Could you check a few things on this model? Use its own coordinates, in mm. A direction names the side the tool comes from. Coordinates: 2 decimals unless noted, no trailing zeros. Order: outer loops, then holes, each group sorted by start corner. A loop starts at its lowest first (then second) coordinate and runs counter-clockwise, first axis right, second up. Notation, with made-up numbers: (13, 4.5) - (37, 4.5) arc R9 ccw to (37, 10.5) - close; hole circle Ø6 at (10, 47). An arc over 180 degrees is marked (long way). Answer as CSV lines item,"result". Start each with the question number.
1. Thinking about a two-plate mould opening in Z: for faces 1 (the face through (-3, 9.5, 3)), 2 (the face through (9.06, 3.94, 6.6)), which applies, released by +Z, released by -Z, zero draft, split by the parting line, or undercut?
2. I want a section at A-A, the plane x = 0. List the corners of the cut face in (y, z) for me, and give its area (3 significant figures).
3. For pin 1 (2.5 mm diameter, centred on x = -5.63, z = -4.95, fed in from +Y); pin 2 (1 mm diameter, centred on x = 5, y = 6, fed in from -Z); pin 3 (2 mm diameter, centred on y = 5, z = -10.5, fed in from -X); pin 4 (5 mm diameter, centred on x = 9, y = 6.5, fed in from +Z), each with a flat end and sliding along its axis, tell me the tip position at first contact or that it passes through.
4. I want a section at C-C, the plane y = 3. Count the separate pieces of the cut face and the enclosed holes in it, and give its area (3 significant figures).
5. I need wall thicknesses on probe 1 along X at (y, z) = (7, 0); probe 2 along Z at (x, y) = (10.75, 6); probe 3 along X at (y, z) = (8.5, -1). Which ranges of each line are inside material? Lowest first, please.
6. I want a section at B-B, the plane z = 0. List the corners of the cut face in (x, y) for me, and give its area (3 significant figures).
7. For faces 3 (the face through (-10, 3.94, 5.07)), 4 (the face through (11.21, 3.94, 0.02)), 5 (the face through (7.21, 4.68, -5.38)), which set-ups out of +Z, -Z, +X, -X, +Y, -Y let a thin tool reach every point of the face, with its end or its side?
from build123d import *

# Parameters (mm, degrees)
BOSS_EXTRUDE1_DEPTH = 8
SKETCH2_R           = 15
BOSS_EXTRUDE2_DEPTH = 1.5
SKETCH4_R           = 4
SKETCH4_R_2         = 1.5
CUT_EXTRUDE1_DEPTH  = 23


with BuildPart() as part:
    # Sketch1 → Boss-Extrude1 (new body)
    with BuildSketch(Plane(origin=(0, 0, 0), x_dir=(1, 0, 0), z_dir=(0, 1, 0))):
        with BuildLine():
            ThreePointArc((-2.619011045, 11.679969227), (-2.794341005, 11.639267947), (-2.969039138, 11.595934917))
            ThreePointArc((-2.969039138, 11.595934917), (-3.464080507, 10.661343548), (-4.413916411, 11.126465832))
            ThreePointArc((-4.413916411, 11.126465832), (-4.580720685, 11.058838004), (-4.746489215, 10.988709666))
            ThreePointArc((-4.746489215, 10.988709666), (-5.089233502, 9.988183136), (-6.100136506, 10.298991922))
            ThreePointArc((-6.100136506, 10.298991922), (-6.25430782, 10.206102767), (-6.407064974, 10.110905915))
            ThreePointArc((-6.407064974, 10.110905915), (-6.589072678, 9.069080507), (-7.636150994, 9.21792265))
            ThreePointArc((-7.636150994, 9.21792265), (-7.773893139, 9.102059408), (-7.909877531, 8.984138103))
            ThreePointArc((-7.909877531, 8.984138103), (-7.926667017, 7.926667017), (-8.984138103, 7.909877531))
            ThreePointArc((-8.984138103, 7.909877531), (-9.102059408, 7.773893139), (-9.21792265, 7.636150994))
            ThreePointArc((-9.21792265, 7.636150994), (-9.069080507, 6.589072678), (-10.110905915, 6.407064974))
            ThreePointArc((-10.110905915, 6.407064974), (-10.206102767, 6.25430782), (-10.298991922, 6.100136506))
            ThreePointArc((-10.298991922, 6.100136506), (-9.988183136, 5.089233502), (-10.988709666, 4.746489215))
            ThreePointArc((-10.988709666, 4.746489215), (-11.058838004, 4.580720685), (-11.126465832, 4.413916411))
            ThreePointArc((-11.126465832, 4.413916411), (-10.661343548, 3.464080507), (-11.595934917, 2.969039138))
            ThreePointArc((-11.595934917, 2.969039138), (-11.639267947, 2.794341005), (-11.679969227, 2.619011045))
            ThreePointArc((-11.679969227, 2.619011045), (-11.071986298, 1.753630353), (-11.917629765, 1.118481464))
            ThreePointArc((-11.917629765, 1.118481464), (-11.933100485, 0.939155376), (-11.945873016, 0.759616935))
            ThreePointArc((-11.945873016, 0.759616935), (-11.21, 0), (-11.945873016, -0.759616935))
            ThreePointArc((-11.945873016, -0.759616935), (-11.933100485, -0.939155376), (-11.917629765, -1.118481464))
            ThreePointArc((-11.917629765, -1.118481464), (-11.071986298, -1.753630353), (-11.679969227, -2.619011045))
            ThreePointArc((-11.679969227, -2.619011045), (-11.639267947, -2.794341005), (-11.595934917, -2.969039138))
            ThreePointArc((-11.595934917, -2.969039138), (-10.661343548, -3.464080507), (-11.126465832, -4.413916411))
            ThreePointArc((-11.126465832, -4.413916411), (-11.058838004, -4.580720685), (-10.988709666, -4.746489215))
            ThreePointArc((-10.988709666, -4.746489215), (-9.988183136, -5.089233502), (-10.298991922, -6.100136506))
            ThreePointArc((-10.298991922, -6.100136506), (-10.206102767, -6.25430782), (-10.110905915, -6.407064974))
            ThreePointArc((-10.110905915, -6.407064974), (-9.069080507, -6.589072678), (-9.21792265, -7.636150994))
            ThreePointArc((-9.21792265, -7.636150994), (-9.102059408, -7.773893139), (-8.984138103, -7.909877531))
            ThreePointArc((-8.984138103, -7.909877531), (-7.926667017, -7.926667017), (-7.909877531, -8.984138103))
            ThreePointArc((-7.909877531, -8.984138103), (-7.773893139, -9.102059408), (-7.636150994, -9.21792265))
            ThreePointArc((-7.636150994, -9.21792265), (-6.589072678, -9.069080507), (-6.407064974, -10.110905915))
            ThreePointArc((-6.407064974, -10.110905915), (-6.25430782, -10.206102767), (-6.100136506, -10.298991922))
            ThreePointArc((-6.100136506, -10.298991922), (-5.089233502, -9.988183136), (-4.746489215, -10.988709666))
            ThreePointArc((-4.746489215, -10.988709666), (-4.580720685, -11.058838004), (-4.413916411, -11.126465832))
            ThreePointArc((-4.413916411, -11.126465832), (-3.464080507, -10.661343548), (-2.969039138, -11.595934917))
            ThreePointArc((-2.969039138, -11.595934917), (-2.794341005, -11.639267947), (-2.619011045, -11.679969227))
            ThreePointArc((-2.619011045, -11.679969227), (-1.753630353, -11.071986298), (-1.118481464, -11.917629765))
            ThreePointArc((-1.118481464, -11.917629765), (-0.939155376, -11.933100485), (-0.759616935, -11.945873016))
            ThreePointArc((-0.759616935, -11.945873016), (0, -11.21), (0.759616935, -11.945873016))
            ThreePointArc((0.759616935, -11.945873016), (0.939155376, -11.933100485), (1.118481464, -11.917629765))
            ThreePointArc((1.118481464, -11.917629765), (1.753630353, -11.071986298), (2.619011045, -11.679969227))
            ThreePointArc((2.619011045, -11.679969227), (2.794341005, -11.639267947), (2.969039138, -11.595934917))
            ThreePointArc((2.969039138, -11.595934917), (3.464080507, -10.661343548), (4.413916411, -11.126465832))
            ThreePointArc((4.413916411, -11.126465832), (4.580720685, -11.058838004), (4.746489215, -10.988709666))
            ThreePointArc((4.746489215, -10.988709666), (5.089233502, -9.988183136), (6.100136506, -10.298991922))
            ThreePointArc((6.100136506, -10.298991922), (6.25430782, -10.206102767), (6.407064974, -10.110905915))
            ThreePointArc((6.407064974, -10.110905915), (6.589072678, -9.069080507), (7.636150994, -9.21792265))
            ThreePointArc((7.636150994, -9.21792265), (7.773893139, -9.102059408), (7.909877531, -8.984138103))
            ThreePointArc((7.909877531, -8.984138103), (7.926667017, -7.926667017), (8.984138103, -7.909877531))
            ThreePointArc((8.984138103, -7.909877531), (9.102059408, -7.773893139), (9.21792265, -7.636150994))
            ThreePointArc((9.21792265, -7.636150994), (9.069080507, -6.589072678), (10.110905915, -6.407064974))
            ThreePointArc((10.110905915, -6.407064974), (10.206102767, -6.25430782), (10.298991922, -6.100136506))
            ThreePointArc((10.298991922, -6.100136506), (9.988183136, -5.089233502), (10.988709666, -4.746489215))
            ThreePointArc((10.988709666, -4.746489215), (11.058838004, -4.580720685), (11.126465832, -4.413916411))
            ThreePointArc((11.126465832, -4.413916411), (10.661343548, -3.464080507), (11.595934917, -2.969039138))
            ThreePointArc((11.595934917, -2.969039138), (11.639267947, -2.794341005), (11.679969227, -2.619011045))
            ThreePointArc((11.679969227, -2.619011045), (11.071986298, -1.753630353), (11.917629765, -1.118481464))
            ThreePointArc((11.917629765, -1.118481464), (11.933100485, -0.939155376), (11.945873016, -0.759616935))
            ThreePointArc((11.945873016, -0.759616935), (11.21, 0), (11.945873016, 0.759616935))
            ThreePointArc((11.945873016, 0.759616935), (11.933100485, 0.939155376), (11.917629765, 1.118481464))
            ThreePointArc((11.917629765, 1.118481464), (11.071986298, 1.753630353), (11.679969227, 2.619011045))
            ThreePointArc((11.679969227, 2.619011045), (11.639267947, 2.794341005), (11.595934917, 2.969039138))
            ThreePointArc((11.595934917, 2.969039138), (10.661343548, 3.464080507), (11.126465832, 4.413916411))
            ThreePointArc((11.126465832, 4.413916411), (11.058838004, 4.580720685), (10.988709666, 4.746489215))
            ThreePointArc((10.988709666, 4.746489215), (9.988183136, 5.089233502), (10.298991922, 6.100136506))
            ThreePointArc((10.298991922, 6.100136506), (10.206102767, 6.25430782), (10.110905915, 6.407064974))
            ThreePointArc((10.110905915, 6.407064974), (9.069080507, 6.589072678), (9.21792265, 7.636150994))
            ThreePointArc((9.21792265, 7.636150994), (9.102059408, 7.773893139), (8.984138103, 7.909877531))
            ThreePointArc((8.984138103, 7.909877531), (7.926667017, 7.926667017), (7.909877531, 8.984138103))
            ThreePointArc((7.909877531, 8.984138103), (7.773893139, 9.102059408), (7.636150994, 9.21792265))
            ThreePointArc((7.636150994, 9.21792265), (6.589072678, 9.069080507), (6.407064974, 10.110905915))
            ThreePointArc((6.407064974, 10.110905915), (6.25430782, 10.206102767), (6.100136506, 10.298991922))
            ThreePointArc((6.100136506, 10.298991922), (5.089233502, 9.988183136), (4.746489215, 10.988709666))
            ThreePointArc((4.746489215, 10.988709666), (4.580720685, 11.058838004), (4.413916411, 11.126465832))
            ThreePointArc((4.413916411, 11.126465832), (3.464080507, 10.661343548), (2.969039138, 11.595934917))
            ThreePointArc((2.969039138, 11.595934917), (2.794341005, 11.639267947), (2.619011045, 11.679969227))
            ThreePointArc((2.619011045, 11.679969227), (1.753630353, 11.071986298), (1.118481464, 11.917629765))
            ThreePointArc((1.118481464, 11.917629765), (0.939155376, 11.933100485), (0.759616935, 11.945873016))
            ThreePointArc((0.759616935, 11.945873016), (0, 11.21), (-0.759616935, 11.945873016))
            ThreePointArc((-0.759616935, 11.945873016), (-0.939155376, 11.933100485), (-1.118481464, 11.917629765))
            ThreePointArc((-1.118481464, 11.917629765), (-1.753630353, 11.071986298), (-2.619011045, 11.679969227))
        make_face()
    extrude(amount=BOSS_EXTRUDE1_DEPTH)

    # Sketch2 → Boss-Extrude2 (add)
    with BuildSketch(Plane(origin=(0, 8, 0), x_dir=(1, 0, 0), z_dir=(0, 1, 0))):
        with Locations(Location((0, 0, 0), (0, 0, 270))):
            Circle(SKETCH2_R)
    extrude(amount=BOSS_EXTRUDE2_DEPTH)

    # Sketch4 → Cut-Extrude1 (cut)
    with BuildSketch(Plane.XZ):
        with Locations(Location((0, 0, 0), (0, 0, 270))):
            Circle(SKETCH4_R)
        with Locations(Location((0, 7.5, 0), (0, 0, 270))):
            Circle(SKETCH4_R_2)
        with Locations(Location((5.944938911, -4.572493996, 0), (0, 0, 270))):
            Circle(SKETCH4_R_2)
        with Locations(Location((-5.630988244, -4.953985406, 0), (0, 0, 270))):
            Circle(SKETCH4_R_2)
    extrude(amount=-CUT_EXTRUDE1_DEPTH, mode=Mode.SUBTRACT)


solid = part.part
Solved:
1,face 1,"zero draft"
1,face 2,"undercut"
2,outline,"(0, -11.21) - (8, -11.21) - (8, -15) - (9.5, -15) - (9.5, -4) - (0, -4) - close; (0, 4) - (9.5, 4) - (9.5, 6) - (0, 6) - close; (0, 9) - (9.5, 9) - (9.5, 15) - (8, 15) - (8, 11.21) - (0, 11.21) - close"
2,area,"120 mm2"
3,pin 1,"passes through"
3,pin 2,"stops at z = -11.09"
3,pin 3,"stops at x = -6.41"
3,pin 4,"stops at z = 13.27"
4,separate pieces,"1"
4,enclosed holes,"4"
4,area,"343 mm2"
5,probe 1,"x = -11.21 to -4, 4 to 11.21"
5,probe 2,"z = -4.68 to -4.12, -3.28 to 3.28, 4.12 to 4.68"
5,probe 3,"x = -14.97 to -3.87, 3.87 to 14.97"
6,outline,"(-15, 8) - (-11.21, 8) - (-11.21, 0) - (-4, 0) - (-4, 9.5) - (-15, 9.5) - close; (4, 0) - (11.21, 0) - (11.21, 8) - (15, 8) - (15, 9.5) - (4, 9.5) - close"
6,area,"148 mm2"
7,face 3,"-Y"
7,face 4,"+X, -Y"
7,face 5,"+Y, -Y"
